Autodesk Inventor part; units mm, degrees
ref_plane "YZ Plane" through (0, 0, 0) normal (1, 0, 0) x (0, 1, 0)
ref_plane "XZ Plane" through (0, 0, 0) normal (0, 1, 0) x (-1, 0, 0)
ref_plane "XY Plane" through (0, 0, 0) normal (0, 0, 1) x (1, 0, 0)
sketch "Sketch1" plane through (0, 0, 0) normal (0, 0, 1) x (1, 0, 0)
  circle A0 centre (0, 0) radius 101.6
  dimension "d0" = 203.2
extrude "Extrusion1" add sketch "Sketch1" along normal mid plane 101.6
sketch "Sketch2" plane through (0, 0, 50.8) normal (0, 0, 1) x (1, 0, 0)
  circle A0 centre (0, 0) radius 101.6
  circle A1 centre (0, 0) radius 101.6
  circle A2 centre (0, 0) radius 38.1
  dimension "d4" = 76.2
extrude "Extrusion2" cut sketch "Sketch2" against normal blind 25.4
mirror "Mirror1" about plane through (0, 0, 0) normal (0, 0, 1) of "Extrusion2"
fillet "Fillet1" radius 12.7 2 edges at (-38.1, 0, 50.8) (-38.1, 0, -50.8)
properties part number "wheel"
Could you check a few things on this model? Use its own coordinates, in mm. A direction names the side the tool comes from. Give positions to 0.01 mm unless a question says otherwise; leave off trailing zeros. Write each loop counter-clockwise with the first axis right and the second up, starting at its lowest first coordinate (ties: lowest second). Pieces come first, ordered by that corner, then holes. Notation, with made-up numbers: (41.25, 48.5) - (97.25, 48.5) arc R18 ccw to (97.25, 55.5) - close; hole circle Ø11 at (-27.5, 12.5). An arc over 180 degrees is marked (long way). Use CSV: the item, a comma, the result in double quotes. Start each with the question number.
Item 1: I want a section at C-C, the plane z = -31. Please give me the cut outline in (x, y), then the cut area to 3 significant figures.
Item 2: I want a section at A-A, the plane y = 0. Please give me the cut outline in (x, z).
Item 3: I'm going to push flat-ended pins straight in: pin 1 (3 mm diameter, centred on y = 46, z = -12.5, fed in from +X); pin 2 (2 mm diameter, centred on x = 18.5, z = -4, fed in from -Y); pin 3 (12 mm diameter, centred on x = 30, z = -26.5, fed in from -Y). Where does each tip first touch, or does it pass through?
Item 4: If I drill on line 1 along Z through (x, y) = (-79.5, -31); line 2 along Y through (x, z) = (-44, -10); line 3 along X through (y, z) = (-14, 43), over which ranges is the centre line in solid material (lowest first)?
Item 5: For faces 1 (the face through (-30.235, -23.183, 31.839)), 2 (the face through (0, 0, 50.8)), 3 (the face through (-44, 1, -25.4)), which set-ups out of +Z, -Z, +X, -X, +Y, -Y let a thin tool reach every point of the face, with its end or its side?
Item 6: I want a section at D-D, the plane z = 0.5. Please give me the cut outline in (x, y), then the cut area to 3 significant figures.
Findings:
1,outline,"circle Ø76.2 at (0, 0)"
1,area,"4,560 mm2"
2,outline,"(-101.6, -25.4) - (-38.1, -25.4) - (-38.1, -38.1) arc R12.7 ccw to (-25.4, -50.8) - (25.4, -50.8) arc R12.7 ccw to (38.1, -38.1) - (38.1, -25.4) - (101.6, -25.4) - (101.6, 25.4) - (38.1, 25.4) - (38.1, 38.1) arc R12.7 ccw to (25.4, 50.8) - (-25.4, 50.8) arc R12.7 ccw to (-38.1, 38.1) - (-38.1, 25.4) - (-101.6, 25.4) - close"
3,pin 1,"stops at x = 91.34"
3,pin 2,"stops at y = -100.08"
3,pin 3,"stops at y = -98.7"
4,line 1,"z = -25.4 to 25.4"
4,line 2,"y = -91.58 to 91.58"
4,line 3,"x = -34.38 to 34.38"
5,face 1,"+Z"
5,face 2,"+Z, +X, -X, +Y, -Y"
5,face 3,"-Z"
6,outline,"circle Ø203.2 at (0, 0)"
6,area,"32,400 mm2"
